Geometry: final body of the model. Coordinates: model frame, mm. Round coordinates to 2 decimals unless told otherwise and drop trailing zeros. Return JSON: item names as keys, results as strings. Group by question number.
1. Draft query along Z for faces 1 (the face through (-0.933, -24.796, -5.506)), 2 (the face through (-0.89, 28.08, 3.69)). Return one class per face: +Z half, -Z half, draft (parallel to the pull), parting line (faces both ways), or undercut.
2. First-contact query: pin 1 Ø8 at (x, z) = (38.5, -12) entering from +Y; pin 2 Ø8 at (y, z) = (6.5, -16.5) entering from +X; pin 3 Ø2 at (x, z) = (9, -14.5) entering from +Y; pin 4 Ø6 at (x, z) = (-35, -5) entering from -Y. Flat tips, straight axial feed; report the tip coordinate or a pass-through.
3. Material intervals for probe 1 along Y at (x, z) = (9, 0); probe 2 along Z at (x, y) = (54, 13.5), sorted ascending.
from build123d import *

# Parameters (mm, degrees)
BOSS_EXTRUDE1_DEPTH      = 66.675
BOSS_EXTRUDE1_DEPTH_BACK = 66.675
SKETCH1_R                = 28.321
F_97_2_DIAMETER_HOLE1_D  = 50.8
CHAMFER1_SIZE            = 2.921


with BuildPart() as part:
    # Sketch1 → Boss-Extrude1 (new, two sides: drawn at the far end of the back side and taken through both)
    with BuildSketch(Plane(origin=(0, 0, 0), x_dir=(0, 0, -1), z_dir=(1, 0, 0)).offset(-BOSS_EXTRUDE1_DEPTH_BACK)):
        Circle(SKETCH1_R)
    extrude(amount=BOSS_EXTRUDE1_DEPTH + BOSS_EXTRUDE1_DEPTH_BACK)

    # #97 (2) Diameter Hole1 (through all)
    with Locations(Plane(origin=(66.675, 0, 0), x_dir=(0, 0, -1), z_dir=(1, 0, 0))):
        with Locations((0, 0)):
            Hole(F_97_2_DIAMETER_HOLE1_D / 2)

    # Chamfer1
    chamfer1_edges = [part.edges().sort_by_distance(p)[0] for p in [
        (66.675, 0, 28.321),
        (-66.675, 0, 28.321),
    ]]
    chamfer(chamfer1_edges, length=CHAMFER1_SIZE - 0.0001)  # a hair under: the kernel refuses the full size


solid = part.part
Taken from the geometry:
{
 "1": {"face 1": "undercut", "face 2": "parting line"},
 "2": {"pin 1": "y = 27.17", "pin 2": "through", "pin 3": "y = 24.9", "pin 4": "y = -28.25"},
 "3": {"probe 1": "-28.32 to -25.4, 25.4 to 28.32", "probe 2": "-24.9 to -21.52, 21.52 to 24.9"}
}
